from build123d import *

# Parameters (mm, degrees)
SKETCH_1_R      = 4
EXTRUDE_1_DEPTH = 23


with BuildPart() as part:
    # Sketch 1 → Extrude 1 (new body)
    with BuildSketch(Plane.XY):
        with BuildLine():
            Line((14, 25.396850198), (14, 35))
            ThreePointArc((14, 35), (0, 49), (-14, 35))
            Line((-14, 35), (-14, 25.396850198))
            ThreePointArc((-14, 25.396850198), (-27.581369596, 8.959243897), (-26.252122851, -12.321771212))
            ThreePointArc((-26.252122851, -12.321771212), (-27.577164466, -27.577164466), (-12.321771212, -26.252122851))
            ThreePointArc((-12.321771212, -26.252122851), (25.83811559, -13.167831361), (14, 25.396850198))
        make_face()
        with BuildLine():
            Line((-7, 18.734993995), (-7, 35))
            ThreePointArc((-7, 35), (0, 42), (7, 35))
            Line((7, 35), (7, 18.734993995))
            ThreePointArc((7, 18.734993995), (0, -20), (-7, 18.734993995))
        make_face(mode=Mode.SUBTRACT)
        with Locations((-20.506096654, -20.506096654)):
            Circle(SKETCH_1_R, mode=Mode.SUBTRACT)
    extrude(amount=EXTRUDE_1_DEPTH)


solid = part.part
Could you check a few things on this model? Use its own coordinates, in mm. A direction names the side the tool comes from. Give positions to 0.01 mm unless a question says otherwise; leave off trailing zeros. Order: outer loops, then holes, each group sorted by start corner. A loop starts at its lowest first (then second) coordinate and runs counter-clockwise, first axis right, second up. Notation, with made-up numbers: (60.25, 73.25) -> (93.25, 73.25) arc R7 ccw to (93.25, 84.25) -> close; hole circle Ø11 at (87, -35.75). An arc over 180 degrees is marked (long way). Answer in a Markdown table with one row per item. Add a question column.
Item 1: Imagine slicing it at B-B (x = 0). List the corners of the cut face in (y, z) for me, and give its area (3 significant figures).
Item 2: Please list where these lines run through material, in increasing order: probe 1 along X at (y, z) = (31, 12.5); probe 2 along X at (y, z) = (0, 10); probe 3 along Y at (x, z) = (-4, 12).
Item 3: Imagine slicing it at A-A (y = 0). List the corners of the cut face in (x, z) for me.
Item 4: For faces 4 (the cylindrical face through (0, 49, 11)), 5 (the flat face through (7, 27, 11)), 6 (the flat face through (14, 30, 11)), which set-ups out of +Z, -Z, +X, -X, +Y, -Y let a thin tool reach every point of the face, with its end or its side?
Item 5: We'd pull the mould along Y, two halves only. Please class faces 1 (the cylindrical face through (25.55, -13.72, 11.34)), 2 (the flat face through (-7, 27, 11)), 3 (the flat face through (-14, 30, 11)): pulls with the +Y half, pulls with the -Y half, needs draft (parallel to the pull), parting line crosses it, or undercut.
Item 6: I'm going to push flat-ended pins straight in: P1, Ø5, axis at x = -8.5, y = -14.5, coming from the +Z side (3 decimals); P2, Ø10, axis at y = -0.5, z = 7.5, coming from the -X side; P3, Ø1, axis at x = 9, z = 4, coming from the +Y side; P4, Ø10.5, axis at y = 28.5, z = 15.5, coming from the -X side. Where does each tip first touch, or does it pass through?
Item 7: Imagine slicing it at C-C (z = 16). List the corners of the cut face in (x, y) for me (3 decimals).
Result:
| question | item | result |
|---|---|---|
| 1 | outline | (-29, 0) -> (-20, 0) -> (-20, 23) -> (-29, 23) -> close; (42, 0) -> (49, 0) -> (49, 23) -> (42, 23) -> close |
| 1 | area | 368 mm2 |
| 2 | probe 1 | -14 to -7, 7 to 14 |
| 2 | probe 2 | -29 to -20, 20 to 29 |
| 2 | probe 3 | -28.72 to -19.6, 40.74 to 48.42 |
| 3 | outline | (-29, 0) -> (-20, 0) -> (-20, 23) -> (-29, 23) -> close; (20, 0) -> (29, 0) -> (29, 23) -> (20, 23) -> close |
| 4 | face 4 | +Z, -Z, +Y |
| 4 | face 5 | +Z, -Z |
| 4 | face 6 | +Z, -Z, +X, +Y |
| 5 | face 1 | parting line crosses it |
| 5 | face 2 | undercut |
| 5 | face 3 | needs draft |
| 6 | P1 | through |
| 6 | P2 | x = -29 |
| 6 | P3 | y = 46.12 |
| 6 | P4 | x = -17.33 |
| 7 | outline | (-26.252, -12.322) arc R10 ccw (long way) to (-12.322, -26.252) arc R29 ccw to (14, 25.397) -> (14, 35) arc R14 ccw to (-14, 35) -> (-14, 25.397) arc R29 ccw to start; hole circle Ø8 at (-20.506, -20.506); hole (-7, 18.735) arc R20 ccw (long way) to (7, 18.735) -> (7, 35) arc R7 ccw to (-7, 35) -> close |
